```python
from build123d import *

# Parameters (mm, degrees)
SKETCH1_W           = 17
SKETCH1_H           = 20
BOSS_EXTRUDE1_DEPTH = 3.15
SKETCH2_W           = 17
SKETCH2_H           = 3.15
BOSS_EXTRUDE2_DEPTH = 16.85
CUT_EXTRUDE1_REACH  = 25.922
SKETCH3_R           = 3
CUT_EXTRUDE2_REACH  = 31.534
SKETCH4_R           = 3
SKETCH4_W           = 6
SKETCH4_H           = 3
BOSS_EXTRUDE3_DEPTH = 2
BOSS_EXTRUDE4_DEPTH = 2


with BuildPart() as part:
    # Sketch1 → Boss-Extrude1 (new body)
    with BuildSketch(Plane(origin=(0, 0, 0), x_dir=(1, 0, 0), z_dir=(0, 1, 0))):
        Rectangle(SKETCH1_W, SKETCH1_H)
    extrude(amount=BOSS_EXTRUDE1_DEPTH)

    # Sketch2 → Boss-Extrude2 (add)
    with BuildSketch(Plane(origin=(0, 3.15, 0), x_dir=(1, 0, 0), z_dir=(0, 1, 0))):
        with Locations((0, 8.425)):
            Rectangle(SKETCH2_W, SKETCH2_H)
    extrude(amount=BOSS_EXTRUDE2_DEPTH)

    # Sketch3 → Cut-Extrude1 (cut, up to next)
    with BuildSketch(Plane.XZ, mode=Mode.PRIVATE) as cut_extrude1_sk1:
        with BuildLine():
            ThreePointArc((-3, -1.5), (0, -4.5), (3, -1.5))
            Line((3, -1.5), (0, -1.5))
            Line((0, -1.5), (-3, -1.5))
        make_face()
    cut_extrude1_tool1 = extrude(cut_extrude1_sk1.sketch, amount=-CUT_EXTRUDE1_REACH, mode=Mode.PRIVATE) & part.part
    # Sketch3 → Cut-Extrude1 (cut, up to next)
    with BuildSketch(Plane.XZ, mode=Mode.PRIVATE) as cut_extrude1_sk2:
        with Locations((0, 1.5)):
            Circle(SKETCH3_R)
    cut_extrude1_tool2 = extrude(cut_extrude1_sk2.sketch, amount=-CUT_EXTRUDE1_REACH, mode=Mode.PRIVATE) & part.part
    # Sketch3 → Cut-Extrude1 (cut, up to next)
    with BuildSketch(Plane.XZ, mode=Mode.PRIVATE) as cut_extrude1_sk3:
        with Locations((0, -1.5)):
            Circle(SKETCH3_R)
    cut_extrude1_tool3 = extrude(cut_extrude1_sk3.sketch, amount=-CUT_EXTRUDE1_REACH, mode=Mode.PRIVATE) & part.part
    # Sketch3 → Cut-Extrude1 (cut, up to next)
    with BuildSketch(Plane.XZ, mode=Mode.PRIVATE) as cut_extrude1_sk4:
        with BuildLine():
            Line((0, -1.5), (3, -1.5))
            ThreePointArc((3, -1.5), (2.897777479, -0.723542865), (2.598076211, 0))
            ThreePointArc((2.598076211, 0), (1.5, -1.098076211), (0, -1.5))
        make_face()
    cut_extrude1_tool4 = extrude(cut_extrude1_sk4.sketch, amount=-CUT_EXTRUDE1_REACH, mode=Mode.PRIVATE) & part.part
    # Sketch3 → Cut-Extrude1 (cut, up to next)
    with BuildSketch(Plane.XZ, mode=Mode.PRIVATE) as cut_extrude1_sk5:
        with BuildLine():
            ThreePointArc((0, -1.5), (-1.5, -1.098076211), (-2.598076211, 0))
            ThreePointArc((-2.598076211, 0), (-2.897777479, -0.723542865), (-3, -1.5))
            Line((-3, -1.5), (0, -1.5))
        make_face()
    cut_extrude1_tool5 = extrude(cut_extrude1_sk5.sketch, amount=-CUT_EXTRUDE1_REACH, mode=Mode.PRIVATE) & part.part
    # Sketch3 → Cut-Extrude1 (cut, up to next)
    with BuildSketch(Plane.XZ, mode=Mode.PRIVATE) as cut_extrude1_sk6:
        with BuildLine():
            ThreePointArc((2.598076211, 0), (2.897777479, 0.723542865), (3, 1.5))
            Line((3, 1.5), (0, 1.5))
            ThreePointArc((0, 1.5), (1.5, 1.098076211), (2.598076211, 0))
        make_face()
    cut_extrude1_tool6 = extrude(cut_extrude1_sk6.sketch, amount=-CUT_EXTRUDE1_REACH, mode=Mode.PRIVATE) & part.part
    # Sketch3 → Cut-Extrude1 (cut, up to next)
    with BuildSketch(Plane.XZ, mode=Mode.PRIVATE) as cut_extrude1_sk7:
        with BuildLine():
            ThreePointArc((-2.598076211, 0), (-1.5, 1.098076211), (0, 1.5))
            Line((0, 1.5), (-3, 1.5))
            ThreePointArc((-3, 1.5), (-2.897777479, 0.723542865), (-2.598076211, 0))
        make_face()
    cut_extrude1_tool7 = extrude(cut_extrude1_sk7.sketch, amount=-CUT_EXTRUDE1_REACH, mode=Mode.PRIVATE) & part.part
    # Sketch3 → Cut-Extrude1 (cut, up to next)
    with BuildSketch(Plane.XZ, mode=Mode.PRIVATE) as cut_extrude1_sk8:
        with BuildLine():
            Line((3, -1.5), (3, 1.5))
            ThreePointArc((3, 1.5), (2.897777479, 0.723542865), (2.598076211, 0))
            ThreePointArc((2.598076211, 0), (2.897777479, -0.723542865), (3, -1.5))
        make_face()
    cut_extrude1_tool8 = extrude(cut_extrude1_sk8.sketch, amount=-CUT_EXTRUDE1_REACH, mode=Mode.PRIVATE) & part.part
    # Sketch3 → Cut-Extrude1 (cut, up to next)
    with BuildSketch(Plane.XZ, mode=Mode.PRIVATE) as cut_extrude1_sk9:
        with BuildLine():
            Line((0, 1.5), (3, 1.5))
            ThreePointArc((3, 1.5), (0, 4.5), (-3, 1.5))
            Line((-3, 1.5), (0, 1.5))
        make_face()
    cut_extrude1_tool9 = extrude(cut_extrude1_sk9.sketch, amount=-CUT_EXTRUDE1_REACH, mode=Mode.PRIVATE) & part.part
    # Sketch3 → Cut-Extrude1 (cut, up to next)
    with BuildSketch(Plane.XZ, mode=Mode.PRIVATE) as cut_extrude1_sk10:
        with BuildLine():
            Line((0, -1.5), (3, -1.5))
            ThreePointArc((3, -1.5), (2.897777479, -0.723542865), (2.598076211, 0))
            ThreePointArc((2.598076211, 0), (1.5, -1.098076211), (0, -1.5))
        make_face()
    cut_extrude1_tool10 = extrude(cut_extrude1_sk10.sketch, amount=-CUT_EXTRUDE1_REACH, mode=Mode.PRIVATE) & part.part
    # Sketch3 → Cut-Extrude1 (cut, up to next)
    with BuildSketch(Plane.XZ, mode=Mode.PRIVATE) as cut_extrude1_sk11:
        with BuildLine():
            ThreePointArc((0, -1.5), (-1.5, -1.098076211), (-2.598076211, 0))
            ThreePointArc((-2.598076211, 0), (-2.897777479, -0.723542865), (-3, -1.5))
            Line((-3, -1.5), (0, -1.5))
        make_face()
    cut_extrude1_tool11 = extrude(cut_extrude1_sk11.sketch, amount=-CUT_EXTRUDE1_REACH, mode=Mode.PRIVATE) & part.part
    # Sketch3 → Cut-Extrude1 (cut, up to next)
    with BuildSketch(Plane.XZ, mode=Mode.PRIVATE) as cut_extrude1_sk12:
        with BuildLine():
            ThreePointArc((-2.598076211, 0), (-2.897777479, 0.723542865), (-3, 1.5))
            Line((-3, 1.5), (-3, -1.5))
            ThreePointArc((-3, -1.5), (-2.897777479, -0.723542865), (-2.598076211, 0))
        make_face()
    cut_extrude1_tool12 = extrude(cut_extrude1_sk12.sketch, amount=-CUT_EXTRUDE1_REACH, mode=Mode.PRIVATE) & part.part
    # Sketch3 → Cut-Extrude1 (cut, up to next)
    with BuildSketch(Plane.XZ, mode=Mode.PRIVATE) as cut_extrude1_sk13:
        with BuildLine():
            ThreePointArc((2.598076211, 0), (2.897777479, 0.723542865), (3, 1.5))
            Line((3, 1.5), (0, 1.5))
            ThreePointArc((0, 1.5), (1.5, 1.098076211), (2.598076211, 0))
        make_face()
    cut_extrude1_tool13 = extrude(cut_extrude1_sk13.sketch, amount=-CUT_EXTRUDE1_REACH, mode=Mode.PRIVATE) & part.part
    # Sketch3 → Cut-Extrude1 (cut, up to next)
    with BuildSketch(Plane.XZ, mode=Mode.PRIVATE) as cut_extrude1_sk14:
        with BuildLine():
            ThreePointArc((-2.598076211, 0), (-1.5, 1.098076211), (0, 1.5))
            Line((0, 1.5), (-3, 1.5))
            ThreePointArc((-3, 1.5), (-2.897777479, 0.723542865), (-2.598076211, 0))
        make_face()
    cut_extrude1_tool14 = extrude(cut_extrude1_sk14.sketch, amount=-CUT_EXTRUDE1_REACH, mode=Mode.PRIVATE) & part.part
    add(cut_extrude1_tool1.solids().sort_by_distance((0, 0, -2.77324))[0], mode=Mode.SUBTRACT)
    add(cut_extrude1_tool2.solids().sort_by_distance((0, 0, 1.5))[0], mode=Mode.SUBTRACT)
    add(cut_extrude1_tool3.solids().sort_by_distance((0, 0, -1.5))[0], mode=Mode.SUBTRACT)
    add(cut_extrude1_tool4.solids().sort_by_distance((2.19025, 0, -1.040207))[0], mode=Mode.SUBTRACT)
    add(cut_extrude1_tool5.solids().sort_by_distance((-2.19025, 0, -1.040207))[0], mode=Mode.SUBTRACT)
    add(cut_extrude1_tool6.solids().sort_by_distance((2.19025, 0, 1.040207))[0], mode=Mode.SUBTRACT)
    add(cut_extrude1_tool7.solids().sort_by_distance((-2.19025, 0, 1.040207))[0], mode=Mode.SUBTRACT)
    add(cut_extrude1_tool8.solids().sort_by_distance((2.880946, 0, 0))[0], mode=Mode.SUBTRACT)
    add(cut_extrude1_tool9.solids().sort_by_distance((0, 0, 2.77324))[0], mode=Mode.SUBTRACT)
    add(cut_extrude1_tool10.solids().sort_by_distance((2.19025, 0, -1.040207))[0], mode=Mode.SUBTRACT)
    add(cut_extrude1_tool11.solids().sort_by_distance((-2.19025, 0, -1.040207))[0], mode=Mode.SUBTRACT)
    add(cut_extrude1_tool12.solids().sort_by_distance((-2.880946, 0, 0))[0], mode=Mode.SUBTRACT)
    add(cut_extrude1_tool13.solids().sort_by_distance((2.19025, 0, 1.040207))[0], mode=Mode.SUBTRACT)
    add(cut_extrude1_tool14.solids().sort_by_distance((-2.19025, 0, 1.040207))[0], mode=Mode.SUBTRACT)

    # Sketch4 → Cut-Extrude2 (cut, up to next)
    with BuildSketch(Plane(origin=(0, 0, -10), x_dir=(-1, 0, 0), z_dir=(0, 0, -1)), mode=Mode.PRIVATE) as cut_extrude2_sk1:
        with Locations((0, 8.5)):
            Circle(SKETCH4_R)
    cut_extrude2_tool1 = extrude(cut_extrude2_sk1.sketch, amount=-CUT_EXTRUDE2_REACH, mode=Mode.PRIVATE) & part.part
    # Sketch4 → Cut-Extrude2 (cut, up to next)
    with BuildSketch(Plane(origin=(0, 0, -10), x_dir=(-1, 0, 0), z_dir=(0, 0, -1)), mode=Mode.PRIVATE) as cut_extrude2_sk2:
        with Locations((0, 11.5)):
            Circle(SKETCH4_R)
    cut_extrude2_tool2 = extrude(cut_extrude2_sk2.sketch, amount=-CUT_EXTRUDE2_REACH, mode=Mode.PRIVATE) & part.part
    # Sketch4 → Cut-Extrude2 (cut, up to next)
    with BuildSketch(Plane(origin=(0, 0, -10), x_dir=(-1, 0, 0), z_dir=(0, 0, -1)), mode=Mode.PRIVATE) as cut_extrude2_sk3:
        with Locations((0, 10)):
            Rectangle(SKETCH4_W, SKETCH4_H)
    cut_extrude2_tool3 = extrude(cut_extrude2_sk3.sketch, amount=-CUT_EXTRUDE2_REACH, mode=Mode.PRIVATE) & part.part
    add(cut_extrude2_tool1.solids().sort_by_distance((0, 8.5, -10))[0], mode=Mode.SUBTRACT)
    add(cut_extrude2_tool2.solids().sort_by_distance((0, 11.5, -10))[0], mode=Mode.SUBTRACT)
    add(cut_extrude2_tool3.solids().sort_by_distance((0, 10, -10))[0], mode=Mode.SUBTRACT)

    # Sketch5 → Boss-Extrude3 (add)
    with BuildSketch(Plane(origin=(8.5, 0, 0), x_dir=(0, 0, -1), z_dir=(1, 0, 0))):
        Polygon((6.85, 20), (-10, 3.15), (6.85, 3.15), align=None)
    extrude(amount=-BOSS_EXTRUDE3_DEPTH)

    # Sketch6 → Boss-Extrude4 (add)
    with BuildSketch(Plane.ZY.offset(8.5)):
        Polygon((10, 3.15), (-6.85, 20), (-6.85, 3.15), align=None)
    extrude(amount=-BOSS_EXTRUDE4_DEPTH)


solid = part.part
```
The model under review builds one solid part; all positions refer to its coordinate system, in mm. A direction names the side the tool comes from. Round coordinates to 2 decimals unless told otherwise and drop trailing zeros. Loops run counter-clockwise (first coordinate to the right, second up) from the corner with the lowest first, then second, coordinate; pieces in that order, holes last. Notation, with made-up numbers: (23.25, 89.5) -> (28.25, 89.5) arc R33 ccw to (28.25, 122.5) -> close; hole circle Ø7 at (-35, 11.5). An arc over 180 degrees is marked (long way). Answer in a Markdown table with one row per item.
1) Consider section A-A, the plane x = 0. Write out the cut boundary in (y, z), plus the area to 3 significant figures.
Taken from the geometry:
| item | result |
|---|---|
| outline | (0, -10) -> (5.5, -10) -> (5.5, -6.85) -> (3.15, -6.85) -> (3.15, -4.5) -> (0, -4.5) -> close; (0, 4.5) -> (3.15, 4.5) -> (3.15, 10) -> (0, 10) -> close; (14.5, -10) -> (20, -10) -> (20, -6.85) -> (14.5, -6.85) -> close |
| area | 59.4 mm² |
2) Draft analysis for pull direction Y (two halves, no side actions). For faces 4 (the flat face through (3, 10, -8)), 5 (the flat face through (-7.51, 11.46, 1.69)), 6 (the flat face through (0, 2, 10)), state which applies: pulls with the +Y half, pulls with the -Y half, needs draft (parallel to the pull), parting line crosses it, or undercut.
Taken from the geometry:
| item | result |
|---|---|
| face 4 | undercut |
| face 5 | pulls with the +Y half |
| face 6 | needs draft |
3) Consider section D-D, the plane z = 5.5. Write out the cut boundary in (x, y), plus the area to 4 significant figures.
Taken from the geometry:
| item | result |
|---|---|
| outline | (-8.5, 0) -> (8.5, 0) -> (8.5, 7.65) -> (6.5, 7.65) -> (6.5, 3.15) -> (-6.5, 3.15) -> (-6.5, 7.65) -> (-8.5, 7.65) -> close |
| area | 71.55 mm² |
4) For pin 1 Ø1.5 at (x, z) = (-1.5, -2.5) entering from +Y; pin 2 Ø3 at (x, y) = (-4, 10) entering from +Z; pin 3 Ø10 at (x, z) = (-0.5, 7.5) entering from +Y, all flat-tipped, find the tip position at first contact; note any pin that passes through.
Taken from the geometry:
| item | result |
|---|---|
| pin 1 | passes through |
| pin 2 | stops at z = -6.85 |
| pin 3 | stops at y = 3.15 |
5) Consider section B-B, the plane z = -1. Write out the cut boundary in (x, y).
Taken from the geometry:
| item | result |
|---|---|
| outline | (-8.5, 0) -> (-3, 0) -> (-3, 3.15) -> (-6.5, 3.15) -> (-6.5, 14.15) -> (-8.5, 14.15) -> close; (3, 0) -> (8.5, 0) -> (8.5, 14.15) -> (6.5, 14.15) -> (6.5, 3.15) -> (3, 3.15) -> close |
6) Consider section C-C, the plane y = 10. Write out the cut boundary in (x, z), plus the area to 4 significant figures.
Taken from the geometry:
| item | result |
|---|---|
| outline | (-8.5, -10) -> (-3, -10) -> (-3, -6.85) -> (-6.5, -6.85) -> (-6.5, 3.15) -> (-8.5, 3.15) -> close; (3, -10) -> (8.5, -10) -> (8.5, 3.15) -> (6.5, 3.15) -> (6.5, -6.85) -> (3, -6.85) -> close |
| area | 74.65 mm² |
7) Wall thickness on line 1 along X through (y, z) = (5.75, -2.75); line 2 along Y through (x, z) = (-3.75, 6); line 3 along Z through (x, y) = (2.25, 4.5): over which ranges is each line inside the solid? List them lowest first.
Taken from the geometry:
| item | result |
|---|---|
| line 1 | x = -8.5 to -6.5, 6.5 to 8.5 |
| line 2 | y = 0 to 3.15 |
| line 3 | z = -10 to -6.85 |
8) Tool access review of faces 1 (the flat face through (6.5, 8, -2)), 2 (the flat face through (-3, 10, -8)), 3 (the flat face through (-3, 2, 0)): name each direction out of +Z, -Z, +X, -X, +Y, -Y from which nothing blocks a thin tool from reaching the whole face with its end or side.
Taken from the geometry:
| item | result |
|---|---|
| face 1 | +Z, +Y |
| face 2 | +Z, -Z |
| face 3 | +Y, -Y |
